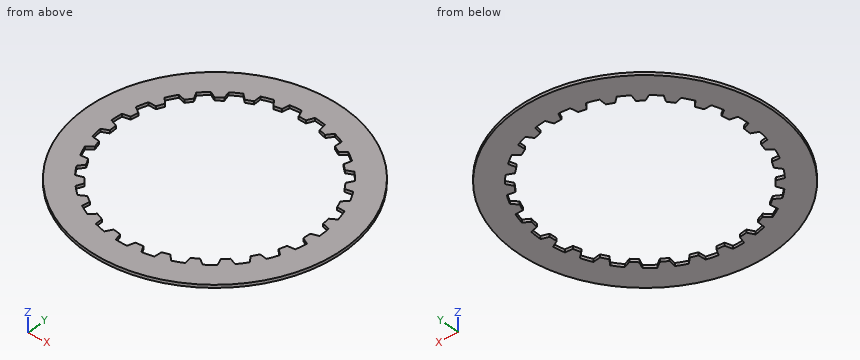
```python
from build123d import *

# Parameters (mm, degrees)
SKETCH1_R           = 66.675
BOSS_EXTRUDE1_DEPTH = 1.524


with BuildPart() as part:
    # Sketch1 → Boss-Extrude1 (new body)
    with BuildSketch(Plane.XY):
        with Locations(Location((0, 0, 0), (0, 0, 180))):
            Circle(SKETCH1_R)
        with BuildLine():
            Line((-3.429, 54.120480412), (-1.905, 50.628557732))
            Line((-1.905, 50.628557732), (1.905, 50.628557732))
            Line((1.905, 50.628557732), (3.429, 54.120480412))
            ThreePointArc((3.429, 54.120480412), (6.29560264, 53.862322902), (9.144470854, 53.452437679))
            Line((9.144470854, 53.452437679), (9.822098447, 49.70318164))
            Line((9.822098447, 49.70318164), (13.529399404, 48.824535172))
            Line((13.529399404, 48.824535172), (15.817612576, 51.870874037))
            ThreePointArc((15.817612576, 51.870874037), (18.547410352, 50.958591133), (21.224960917, 49.902760195))
            Line((21.224960917, 49.902760195), (21.019685025, 46.09829416))
            Line((21.019685025, 46.09829416), (24.424425385, 44.388369284))
            Line((24.424425385, 44.388369284), (27.353493565, 46.824895417))
            ThreePointArc((27.353493565, 46.824895417), (29.799322372, 45.307668525), (32.161207844, 43.662811992))
            Line((32.161207844, 43.662811992), (31.084094942, 40.00823571))
            Line((31.084094942, 40.00823571), (34.002724271, 37.559214917))
            Line((34.002724271, 37.559214917), (37.414740634, 39.254574565))
            ThreePointArc((37.414740634, 39.254574565), (39.444745209, 37.21419778), (41.36363573, 35.068990293))
            Line((41.36363573, 35.068990293), (39.472753256, 31.761322918))
            Line((39.472753256, 31.761322918), (41.74792749, 28.705233553))
            Line((41.74792749, 28.705233553), (45.458949352, 29.568029437))
            ThreePointArc((45.458949352, 29.568029437), (46.963691622, 27.1145), (48.336139308, 24.58459025))
            Line((48.336139308, 24.58459025), (45.733425224, 21.802148985))
            Line((45.733425224, 21.802148985), (47.242489132, 18.303745618))
            Line((47.242489132, 18.303745618), (51.052454344, 18.287464189))
            ThreePointArc((51.052454344, 18.287464189), (51.950813263, 15.553052507), (52.702829105, 12.774828583))
            Line((52.702829105, 12.774828583), (49.5285964, 10.667615558))
            Line((49.5285964, 10.667615558), (50.190195957, 6.915498019))
            Line((50.190195957, 6.915498019), (53.893708307, 6.021017013))
            ThreePointArc((53.893708307, 6.021017013), (54.137253115, 3.153135927), (54.228295743, 0.276372601))
            Line((54.228295743, 0.276372601), (50.653668125, -1.042011786))
            Line((50.653668125, -1.042011786), (50.432136326, -4.845565869))
            Line((50.432136326, -4.845565869), (53.829538506, -6.570024749))
            ThreePointArc((53.829538506, -6.570024749), (53.405139638, -9.416767027), (52.830300921, -12.2369827))
            Line((52.830300921, -12.2369827), (49.047987489, -12.695464004))
            Line((49.047987489, -12.695464004), (47.955267173, -16.345404046))
            Line((47.955267173, -16.345404046), (50.863404351, -18.806874776))
            ThreePointArc((50.863404351, -18.806874776), (49.79394126, -21.479009633), (48.584210902, -24.090639096))
            Line((48.584210902, -24.090639096), (44.798117153, -23.664500472))
            Line((44.798117153, -23.664500472), (42.893117153, -26.96405726))
            Line((42.893117153, -26.96405726), (45.155210902, -30.029841315))
            ThreePointArc((45.155210902, -30.029841315), (43.49833862, -32.383313269), (41.718933497, -34.645562903))
            Line((41.718933497, -34.645562903), (38.133168725, -33.357777594))
            Line((38.133168725, -33.357777594), (35.518588085, -36.129071168))
            Line((35.518588085, -36.129071168), (37.012688345, -39.633891337))
            ThreePointArc((37.012688345, -39.633891337), (34.857729286, -41.541824106), (32.604577589, -43.332735446))
            Line((32.604577589, -43.332735446), (29.412451301, -41.252728291))
            Line((29.412451301, -41.252728291), (26.22924274, -43.346357498))
            Line((26.22924274, -43.346357498), (26.874802178, -47.101268018))
            ThreePointArc((26.874802178, -47.101268018), (24.337930743, -48.460804452), (21.732500464, -49.683829005))
            Line((21.732500464, -49.683829005), (19.106101015, -46.923733729))
            Line((19.106101015, -46.923733729), (15.525872129, -48.226830475))
            Line((15.525872129, -48.226830475), (15.288088471, -52.029403148))
            ThreePointArc((15.288088471, -52.029403148), (12.506068054, -52.767250287), (9.688818614, -53.356454482))
            Line((9.688818614, -53.356454482), (7.769735877, -50.065068535))
            Line((7.769735877, -50.065068535), (3.985497734, -50.507382538))
            Line((3.985497734, -50.507382538), (2.877189956, -54.152619687))
            ThreePointArc((2.877189956, -54.152619687), (0, -54.229), (-2.877189956, -54.152619687))
            Line((-2.877189956, -54.152619687), (-3.985497734, -50.507382538))
            Line((-3.985497734, -50.507382538), (-7.769735877, -50.065068535))
            Line((-7.769735877, -50.065068535), (-9.688818614, -53.356454482))
            ThreePointArc((-9.688818614, -53.356454482), (-12.506068054, -52.767250287), (-15.288088471, -52.029403148))
            Line((-15.288088471, -52.029403148), (-15.525872129, -48.226830475))
            Line((-15.525872129, -48.226830475), (-19.106101015, -46.923733729))
            Line((-19.106101015, -46.923733729), (-21.732500464, -49.683829005))
            ThreePointArc((-21.732500464, -49.683829005), (-24.337930743, -48.460804452), (-26.874802178, -47.101268018))
            Line((-26.874802178, -47.101268018), (-26.22924274, -43.346357498))
            Line((-26.22924274, -43.346357498), (-29.412451301, -41.252728291))
            Line((-29.412451301, -41.252728291), (-32.604577589, -43.332735446))
            ThreePointArc((-32.604577589, -43.332735446), (-34.857729286, -41.541824106), (-37.012688345, -39.633891337))
            Line((-37.012688345, -39.633891337), (-35.518588085, -36.129071168))
            Line((-35.518588085, -36.129071168), (-38.133168725, -33.357777594))
            Line((-38.133168725, -33.357777594), (-41.718933497, -34.645562903))
            ThreePointArc((-41.718933497, -34.645562903), (-43.49833862, -32.383313269), (-45.155210902, -30.029841315))
            Line((-45.155210902, -30.029841315), (-42.893117153, -26.96405726))
            Line((-42.893117153, -26.96405726), (-44.798117153, -23.664500472))
            Line((-44.798117153, -23.664500472), (-48.584210902, -24.090639096))
            ThreePointArc((-48.584210902, -24.090639096), (-49.79394126, -21.479009633), (-50.863404351, -18.806874776))
            Line((-50.863404351, -18.806874776), (-47.955267173, -16.345404046))
            Line((-47.955267173, -16.345404046), (-49.047987489, -12.695464004))
            Line((-49.047987489, -12.695464004), (-52.830300921, -12.2369827))
            ThreePointArc((-52.830300921, -12.2369827), (-53.405139638, -9.416767027), (-53.829538506, -6.570024749))
            Line((-53.829538506, -6.570024749), (-50.432136326, -4.845565869))
            Line((-50.432136326, -4.845565869), (-50.653668125, -1.042011786))
            Line((-50.653668125, -1.042011786), (-54.228295743, 0.276372601))
            ThreePointArc((-54.228295743, 0.276372601), (-54.137253115, 3.153135927), (-53.893708307, 6.021017013))
            Line((-53.893708307, 6.021017013), (-50.190195957, 6.915498019))
            Line((-50.190195957, 6.915498019), (-49.5285964, 10.667615558))
            Line((-49.5285964, 10.667615558), (-52.702829105, 12.774828583))
            ThreePointArc((-52.702829105, 12.774828583), (-51.950813263, 15.553052507), (-51.052454344, 18.287464189))
            Line((-51.052454344, 18.287464189), (-47.242489132, 18.303745618))
            Line((-47.242489132, 18.303745618), (-45.733425224, 21.802148985))
            Line((-45.733425224, 21.802148985), (-48.336139308, 24.58459025))
            ThreePointArc((-48.336139308, 24.58459025), (-46.963691622, 27.1145), (-45.458949352, 29.568029437))
            Line((-45.458949352, 29.568029437), (-41.74792749, 28.705233553))
            Line((-41.74792749, 28.705233553), (-39.472753256, 31.761322918))
            Line((-39.472753256, 31.761322918), (-41.36363573, 35.068990293))
            ThreePointArc((-41.36363573, 35.068990293), (-39.444745209, 37.21419778), (-37.414740634, 39.254574565))
            Line((-37.414740634, 39.254574565), (-34.002724271, 37.559214917))
            Line((-34.002724271, 37.559214917), (-31.084094942, 40.00823571))
            Line((-31.084094942, 40.00823571), (-32.161207844, 43.662811992))
            ThreePointArc((-32.161207844, 43.662811992), (-29.799322372, 45.307668525), (-27.353493565, 46.824895417))
            Line((-27.353493565, 46.824895417), (-24.424425385, 44.388369284))
            Line((-24.424425385, 44.388369284), (-21.019685025, 46.09829416))
            Line((-21.019685025, 46.09829416), (-21.224960917, 49.902760195))
            ThreePointArc((-21.224960917, 49.902760195), (-18.547410352, 50.958591133), (-15.817612576, 51.870874037))
            Line((-15.817612576, 51.870874037), (-13.529399404, 48.824535172))
            Line((-13.529399404, 48.824535172), (-9.822098447, 49.70318164))
            Line((-9.822098447, 49.70318164), (-9.144470854, 53.452437679))
            ThreePointArc((-9.144470854, 53.452437679), (-6.29560264, 53.862322902), (-3.429, 54.120480412))
        make_face(mode=Mode.SUBTRACT)
    extrude(amount=BOSS_EXTRUDE1_DEPTH)


solid = part.part
```
CAD build for the part. Positions are in the model's coordinates, mm. Coordinates: 2 decimals unless noted, no trailing zeros. Order: outer loops, then holes, each group sorted by start corner. A loop starts at its lowest first (then second) coordinate and runs counter-clockwise, first axis right, second up. Notation, with made-up numbers: (-20.75, -13.75) - (-14.75, -13.75) arc R29 cw to (-14.75, 14.25) - close; hole circle Ø11 at (38.25, -5.75). An arc over 180 degrees is marked (long way). Use a Markdown table: item, result. Add a question column.
(1) Flat gauge pins, fed straight in: pin 1 (12 mm diameter, centred on x = 38.5, y = 12.5, fed in from +Z) (3 decimals); pin 2 (0.8 mm diameter, centred on x = -0.5, z = 0.5, fed in from -Y). Where does each tip first touch, or does it go through?
(2) Saw through at A-A (x = 0). Give the cut face in (y, z) (3 decimals).
(3) Drill centre lines: line 1 along X through (y, z) = (45, 0.4); line 2 along X through (y, z) = (50, 0.6); line 3 along X through (y, z) = (-32.5, 0.9). Where is each one in solid material? Low to high. Write a range as [from, to].
Solved:
| question | item | result |
|---|---|---|
| 1 | pin 1 | passes through |
| 1 | pin 2 | stops at y = -66.67 |
| 2 | outline | (-66.675, 0) - (-54.229, 0) - (-54.229, 1.524) - (-66.675, 1.524) - close; (50.629, 0) - (66.675, 0) - (66.675, 1.524) - (50.629, 1.524) - close |
| 3 | line 1 | x = [-49.2, -30.26], [-25.16, -23.21], [23.21, 25.16], [30.26, 49.2] |
| 3 | line 2 | x = [-44.11, -20.99], [-14.41, -9.77], [9.77, 14.41], [20.99, 44.11] |
| 3 | line 3 | x = [-58.22, -43.41], [43.41, 58.22] |
